from build123d import *

# Parameters (mm, degrees)
F1_DEPTH = 101.6
F3_D     = 5.5
F5_D     = 3.7973


with BuildPart() as f1:
    # F0 (on Right) → F1 (new body)
    with BuildSketch(Plane.YZ):
        Polygon((-19.05, -3.175), (19.05, -3.175), (19.05, 3.175), (12.7, 3.175), (-19.05, 3.175), align=None)
        with BuildLine():
            Line((12.7, 3.175), (19.05, 3.175))
            Line((19.05, 3.175), (19.05, 35.775738686))
            ThreePointArc((19.05, 35.775738686), (15.875, 34.925), (12.7, 35.775738686))
            Line((12.7, 35.775738686), (12.7, 3.175))
        make_face()
        with BuildLine():
            ThreePointArc((12.7, 35.775738686), (15.875, 34.925), (19.05, 35.775738686))
            Line((19.05, 35.775738686), (19.05, 41.275))
            Line((19.05, 41.275), (12.7, 41.275))
            Line((12.7, 41.275), (12.7, 35.775738686))
        make_face()
        with BuildLine():
            Line((19.05, 41.275), (19.05, 35.775738686))
            ThreePointArc((19.05, 35.775738686), (21.374261314, 38.1), (22.225, 41.275))
            ThreePointArc((22.225, 41.275), (12.7, 46.774261314), (12.7, 35.775738686))
            Line((12.7, 35.775738686), (12.7, 41.275))
            Line((12.7, 41.275), (19.05, 41.275))
        make_face()
    extrude(amount=F1_DEPTH)

    # F3 (through all)
    with Locations(Plane(origin=(0, 0, 0), x_dir=(0, 1, 0), z_dir=(-1, 0, 0))):
        with Locations((15.6024256721, -41.1942079663)):
            Hole(F3_D / 2)

    # F5 (through all)
    with Locations(Plane.XY.offset(3.175)):
        with Locations((14.0319131315, -8.2768965513), (81.3887268305, -9.2282639816), (84.8136544228, -9.2282639816)):
            Hole(F5_D / 2)


solid = f1.part
Work out the finished part from the listing and answer in its coordinate system (mm). A direction names the side the tool comes from. Give positions to 0.01 mm unless a question says otherwise; leave off trailing zeros. Loops run counter-clockwise (first coordinate to the right, second up) from the corner with the lowest first, then second, coordinate; pieces in that order, holes last. Notation, with made-up numbers: (11, -30) -> (52, -30) arc R18 cw to (52, -6) -> close; hole circle Ø1 at (43.25, 49). An arc over 180 degrees is marked (long way). Use a Markdown table: item, result. Add a question column.
1. Flat-ended cylindrical pins translate along their axes: pin 1 Ø2.5 at (x, y) = (84.81, -9.23) entering from -Z; pin 2 Ø10 at (x, z) = (61.5, 25.5) entering from -Y; pin 3 Ø8 at (x, z) = (80.5, 35) entering from +Y; pin 4 Ø6 at (y, z) = (16, 25.5) entering from -X. Find the tip coordinate at first contact, or state that the pin passes through.
2. Find the intervals of material crossed by probe 1 along Y at (x, z) = (94, 12); probe 2 along Z at (x, y) = (4.5, 11) (3 decimals); probe 3 along Z at (x, y) = (70, 0) (3 decimals), in increasing order.
3. For faces 4 (the flat face through (0, 14, 17)), 5 (the flat face through (50, 19.05, 16)), determine the directions among +Z, -Z, +X, -X, +Y, -Y from which every point of the face is accessible in a straight line to the end or side of a thin tool.
4. Section A-A on z = 5 is taken. Determine the outline of the cut face in (x, y).
5. Determine the mould class of faces 1 (the cylindrical face through (51.511, 15.96, 38.468)), 2 (the flat face through (50, 0, -3.175)), 3 (the flat face through (50, 12.7, 20)) for opening direction Y: released by +Y, released by -Y, zero draft, split by the parting line, or undercut.
6. Section B-B on x = 26 is taken. Determine the outline of the cut face in (y, z) (3 decimals), and give its area (3 significant figures).
7. Section C-C on y = 5 is taken. Determine the outline of the cut face in (x, z) (3 decimals), and give its area (3 significant figures).
Results below:
| question | item | result |
|---|---|---|
| 1 | pin 1 | passes through |
| 1 | pin 2 | stops at y = 12.7 |
| 1 | pin 3 | stops at y = 21.8 |
| 1 | pin 4 | stops at x = 0 |
| 2 | probe 1 | y = 12.7 to 19.05 |
| 2 | probe 2 | z = -3.175 to 3.175, 37.206 to 45.344 |
| 2 | probe 3 | z = -3.175 to 3.175 |
| 3 | face 4 | +Z, -Z, -X, +Y, -Y |
| 3 | face 5 | -Z, +X, -X, +Y |
| 4 | outline | (0, 12.7) -> (101.6, 12.7) -> (101.6, 19.05) -> (0, 19.05) -> close |
| 5 | face 1 | undercut |
| 5 | face 2 | zero draft |
| 5 | face 3 | released by -Y |
| 6 | outline | (-19.05, -3.175) -> (19.05, -3.175) -> (19.05, 35.776) arc R6.35 ccw (long way) to (12.7, 35.776) -> (12.7, 3.175) -> (-19.05, 3.175) -> close; hole circle Ø5.5 at (15.602, 41.194) |
| 6 | area | 548 mm^2 |
| 7 | outline | (0, -3.175) -> (101.6, -3.175) -> (101.6, 3.175) -> (0, 3.175) -> close |
| 7 | area | 645 mm^2 |
